```python
from build123d import *

# Parameters (mm, degrees)
SKETCH_1_R          = 4.75
EXTRUDE_1_DEPTH     = 30
SKETCH_2_R          = 2.75
CUT_EXTRUDE_1_DEPTH = 0.5
SKETCH_3_R          = 2.5
EXTRUDE_2_DEPTH     = 22.5
EXTRUDE_START       = 0.5
SKETCH_4_R          = 2.5
EXTRUDE_3_DEPTH     = 0.5
CUT_EXTRUDE_START   = -22.5
CUT_EXTRUDE_2_DEPTH = 22.5


with BuildPart() as part:
    # 草图1 → 凸台-拉伸1 (new body)
    with BuildSketch(Plane(origin=(0, 0, 0), x_dir=(1, 0, 0), z_dir=(0, 1, 0))):
        with Locations(Location((0, 0, 0), (0, 0, 270))):
            Circle(SKETCH_1_R)
    extrude(amount=EXTRUDE_1_DEPTH)

    # 草图2 → 切除-拉伸1 (cut)
    with BuildSketch(Plane(origin=(0, 30, 0), x_dir=(1, 0, 0), z_dir=(0, 1, 0))):
        with Locations(Location((0, 0, 0), (0, 0, 270))):
            Circle(SKETCH_2_R)
    extrude(amount=-CUT_EXTRUDE_1_DEPTH, mode=Mode.SUBTRACT)

    # 草图3 → 凸台-拉伸2 (add)
    with BuildSketch(Plane(origin=(0, 29.5, 0), x_dir=(1, 0, 0), z_dir=(0, 1, 0))):
        with Locations(Location((0, 0, 0), (0, 0, 90))):
            Circle(SKETCH_3_R)
    extrude(amount=EXTRUDE_2_DEPTH)

    # 草图4 → 凸台-拉伸3 (add)
    with BuildSketch(Plane.XZ.offset(EXTRUDE_START)):
        with Locations(Location((0, 0, 0), (0, 0, 270))):
            Circle(SKETCH_4_R)
    extrude(amount=-EXTRUDE_3_DEPTH)

    # 草图5 → 切除-拉伸2 (cut)
    with BuildSketch(Plane(origin=(0, 52, 0), x_dir=(1, 0, 0), z_dir=(0, 1, 0)).offset(CUT_EXTRUDE_START)):
        with BuildLine():
            Line((1.5, -2), (-1.5, -2))
            ThreePointArc((-1.5, -2), (0, -2.5), (1.5, -2))
        make_face()
    extrude(amount=CUT_EXTRUDE_2_DEPTH, mode=Mode.SUBTRACT)


solid = part.part
```
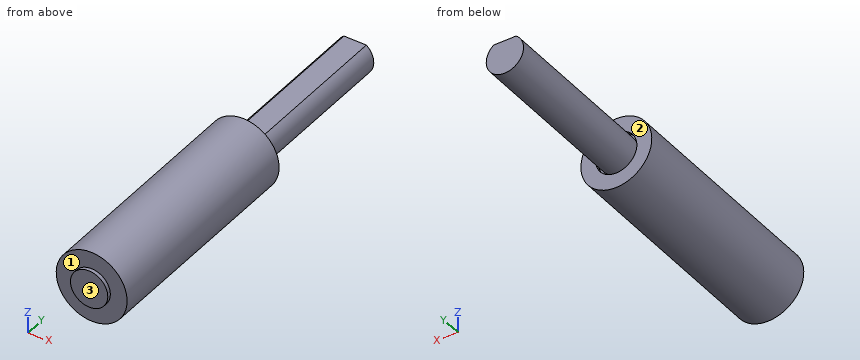
Input: part model. Units: mm. Frame: model coordinates. Face numbers are marked on the shaded views. A direction names the side the tool comes from. Coordinates: 2 decimals unless noted, no trailing zeros. Loops run counter-clockwise (first coordinate to the right, second up) from the corner with the lowest first, then second, coordinate; pieces in that order, holes last. Notation, with made-up numbers: M -3,31 L 54,31 A23 ccw 54,65 Z; hole C -18,20.25 d4. An arc over 180 degrees is marked long. Use a Markdown table: item, result. Add a question column.
1) Section D-D, the plane y = 3. Return the cut outline in (x, z).
2) Section A-A, the plane z = 0. Return the cut outline in (x, y).
3) Section B-B, the plane x = 0. Return the cut outline in (y, z), plus the area to 3 significant figures.
4) Pin query (flat end, axial travel): P1, Ø1.5, axis at y = 20.5, z = 2, coming from the -X side; P2, Ø1.5, axis at y = 37, z = 3, coming from the +X side; P3, Ø1.5, axis at y = 18.5, z = 2.5, coming from the +X side; P4, Ø1.5, axis at y = 16, z = 1.5, coming from the -X side. Return the tip coordinate at first contact, or that it passes through.
5) Section C-C, the plane y = 38.5. Return the cut outline in (x, z).
6) Line query: L1, parallel to X at y = 29.75, z = 0; L2, parallel to Y at x = 3.5, z = 2.5; L3, parallel to X at y = 26, z = -0.25. Output: solid intervals per line, ascending. Write a range as from..to.
7) Set-up query: the marked faces 1, 2 and 3. Return all of +Z, -Z, +X, -X, +Y, -Y with unobstructed straight access to the full face (end or side cutting, diameter ignored); none if empty.
Answer below:
| question | item | result |
|---|---|---|
| 1 | outline | C 0,0 d9.5 |
| 2 | outline | M -4.75,0 L -2.5,0 L -2.5,-0.5 L 2.5,-0.5 L 2.5,0 L 4.75,0 L 4.75,30 L 2.75,30 L 2.75,29.5 L 2.5,29.5 L 2.5,52 L -2.5,52 L -2.5,29.5 L -2.75,29.5 L -2.75,30 L -4.75,30 Z |
| 3 | outline | M -0.5,-2.5 L 0,-2.5 L 0,-4.75 L 30,-4.75 L 30,-2.75 L 29.5,-2.75 L 29.5,-2.5 L 52,-2.5 L 52,2 L 29.5,2 L 29.5,2.75 L 30,2.75 L 30,4.75 L 0,4.75 L 0,2.5 L -0.5,2.5 Z |
| 3 | area | 386 mm2 |
| 4 | P1 | x = -4.58 |
| 4 | P2 | through |
| 4 | P3 | x = 4.42 |
| 4 | P4 | x = -4.69 |
| 5 | outline | M -1.5,2 A2.5 ccw long 1.5,2 Z |
| 6 | L1 | -4.75..-2.75, -2.5..2.5, 2.75..4.75 |
| 6 | L2 | 0..30 |
| 6 | L3 | -4.74..4.74 |
| 7 | face 1 | -Y |
| 7 | face 2 | +Y |
| 7 | face 3 | +Z, -Z, +X, -X, -Y |
